```python
from build123d import *

# Parameters (mm, degrees)
BOSS_EXTRUDE1_DEPTH = 3
BOSS_EXTRUDE2_DEPTH = 3
FILLET1_R           = 4
LPATTERN1_COUNT     = 5
LPATTERN1_PITCH     = 30.4
SKETCH5_W           = 158.4
SKETCH5_H           = 3
BOSS_EXTRUDE3_DEPTH = 15
SKETCH6_W           = 25
SKETCH6_H           = 7
CUT_EXTRUDE1_DEPTH  = 60
SKETCH7_W           = 61.7
SKETCH7_H           = 13.2
CUT_EXTRUDE2_DEPTH  = 10
FILLET2_R           = 10


with BuildPart() as part:
    # Sketch1 → Boss-Extrude1 (new body)
    with BuildSketch(Plane(origin=(0, 0, 0), x_dir=(1, 0, 0), z_dir=(0, 1, 0))):
        Polygon((26, -9.073446812), (-10.8, -9.073446812), (-10.8, -5.873446812), (-10.8, 5.126553188), (-4.4, 5.126553188), (-4.4, -5.873446812), (4.4, -5.873446812), (4.4, 5.126553188), (10.798731059, 5.126553188), (10.798731059, -5.873446812), (19.6, -5.873446812), (19.6, 5.126553188), (26, 5.126553188), align=None)
    extrude(amount=BOSS_EXTRUDE1_DEPTH)

    # Sketch2 → Boss-Extrude2 (add)
    with BuildSketch(Plane(origin=(0, 3, 0), x_dir=(1, 0, 0), z_dir=(0, 1, 0))):
        Polygon((-10.8, 5.126553188), (-7.6, 11.126553188), (-4.4, 5.126553188), align=None)
        Polygon((4.4, 5.126553188), (7.59936553, 11.126553188), (10.798731059, 5.126553188), align=None)
        Polygon((19.6, 5.126553188), (22.8, 11.126553188), (26, 5.126553188), align=None)
    extrude(amount=-BOSS_EXTRUDE2_DEPTH)

    # Fillet1
    fillet1_edges = [part.edges().sort_by_distance(p)[0] for p in [
        (-4.4, 1.5, 5.873446812),
        (4.4, 1.5, 5.873446812),
        (10.798731059, 1.5, 5.873446812),
        (19.6, 1.5, 5.873446812),
    ]]
    fillet(fillet1_edges, radius=FILLET1_R)


with BuildPart() as lpattern1_1:
    # LPattern1: pattern copy
    add(part.part.moved(Location(Vector(1, 0, 0) * (1 * LPATTERN1_PITCH))))


with BuildPart() as lpattern1_2:
    # LPattern1: pattern copy
    add(part.part.moved(Location(Vector(1, 0, 0) * (2 * LPATTERN1_PITCH))))


with BuildPart() as lpattern1_3:
    # LPattern1: pattern copy
    add(part.part.moved(Location(Vector(1, 0, 0) * (3 * LPATTERN1_PITCH))))


with BuildPart() as lpattern1_4:
    # LPattern1: pattern copy
    add(part.part.moved(Location(Vector(1, 0, 0) * (4 * LPATTERN1_PITCH))))


with BuildPart() as part_1:
    add(part.part)

    # Combine1: union LPattern1_1, LPattern1_2, LPattern1_3, LPattern1_4
    add(lpattern1_1.part)
    add(lpattern1_2.part)
    add(lpattern1_3.part)
    add(lpattern1_4.part)

    # Sketch5 → Boss-Extrude3 (add)
    with BuildSketch(Plane.XY.offset(9.073446812)):
        with Locations((68.4, 1.5)):
            Rectangle(SKETCH5_W, SKETCH5_H)
    extrude(amount=BOSS_EXTRUDE3_DEPTH)

    # Sketch6 → Cut-Extrude1 (cut)
    with BuildSketch(Plane(origin=(0, 3, 0), x_dir=(1, 0, 0), z_dir=(0, 1, 0))):
        with Locations((68.4, -15.573446812)):
            Rectangle(SKETCH6_W, SKETCH6_H)
    extrude(amount=-CUT_EXTRUDE1_DEPTH, mode=Mode.SUBTRACT)

    # Sketch7 → Cut-Extrude2 (cut)
    with BuildSketch(Plane(origin=(0, 3, 0), x_dir=(1, 0, 0), z_dir=(0, 1, 0))):
        with Locations((20.05, -17.473446812)):
            Rectangle(SKETCH7_W, SKETCH7_H)
        with Locations((116.75, -17.473446812)):
            Rectangle(SKETCH7_W, SKETCH7_H)
    extrude(amount=-CUT_EXTRUDE2_DEPTH, mode=Mode.SUBTRACT)

    # Fillet2
    fillet2_edges = [part_1.edges().sort_by_distance(p)[0] for p in [
        (50.9, 1.5, 10.873446812),
        (85.9, 1.5, 10.873446812),
    ]]
    fillet(fillet2_edges, radius=FILLET2_R)


solid = part_1.part
```
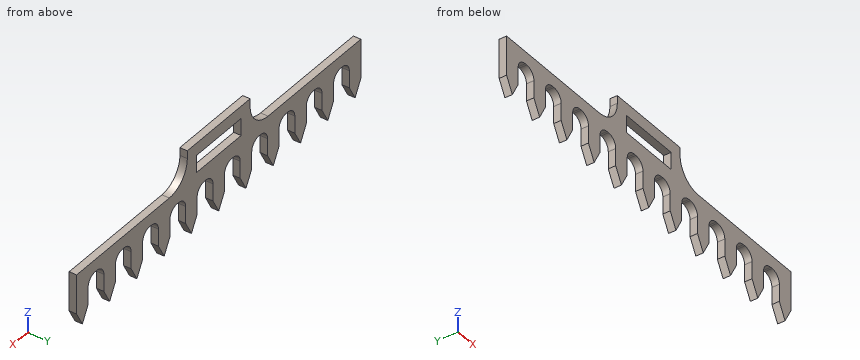
Read the model definition and answer for the solid it produces. Units are mm, in the model's axes. Give positions to 0.01 mm unless a question says otherwise; leave off trailing zeros. Loops run counter-clockwise (first coordinate to the right, second up) from the corner with the lowest first, then second, coordinate; pieces in that order, holes last.
Item 1: The part is cut by section A-A (z = 16). Write down the section's boundary in (x, y), and give its area (3 significant figures).
Item 2: Find the intervals of material crossed by line 1 along Z through (x, y) = (69.5, 0.7); line 2 along X through (y, z) = (1.5, 22.5); line 3 along Z through (x, y) = (62.5, 2.85), in increasing order.
Item 3: Each of these flat-tipped pins is pushed along its axis until it touches: pin 1 Ø10 at (x, z) = (126, 20.5) entering from -Y; pin 2 Ø0.9 at (x, y) = (60.5, 1.5) entering from -Z; pin 3 Ø1.5 at (x, y) = (89, 1.5) entering from -Z; pin 4 Ø1 at (y, z) = (2, 15.5) entering from -X. Where does it stop, or does it pass through?
Item 4: The part is cut by section B-B (z = 3.5). Give the number of separate pieces and of enclosed holes in the cut face, and give its area (3 significant figures).
Taken from the geometry:
1. outline: (49.63, 0) - (55.9, 0) - (55.9, 3) - (49.63, 3) - close; (80.9, 0) - (87.17, 0) - (87.17, 3) - (80.9, 3) - close
1. area: 37.6 mm2
2. line 1: z = -9.06 to 12.07, 19.07 to 24.07
2. line 2: x = 50.9 to 85.9
2. line 3: z = 5.66 to 12.07, 19.07 to 24.07
3. pin 1: passes through
3. pin 2: stops at z = 5.86
3. pin 3: stops at z = 4.96
3. pin 4: stops at x = 48.99
4. separate pieces: 11
4. enclosed holes: 0
4. area: 232 mm2
